Input: part model. Units: mm. Frame: model coordinates. Face numbers are marked on the shaded views. Round coordinates to 2 decimals unless told otherwise and drop trailing zeros. Order: outer loops, then holes, each group sorted by start corner. A loop starts at its lowest first (then second) coordinate and runs counter-clockwise, first axis right, second up. Notation, with made-up numbers: (-30.75, -10.5) -> (8.25, -10.5) arc R20 ccw to (8.25, -2.5) -> close; hole circle Ø9 at (-17, 66.25). An arc over 180 degrees is marked (long way). Use a Markdown table: item, result.
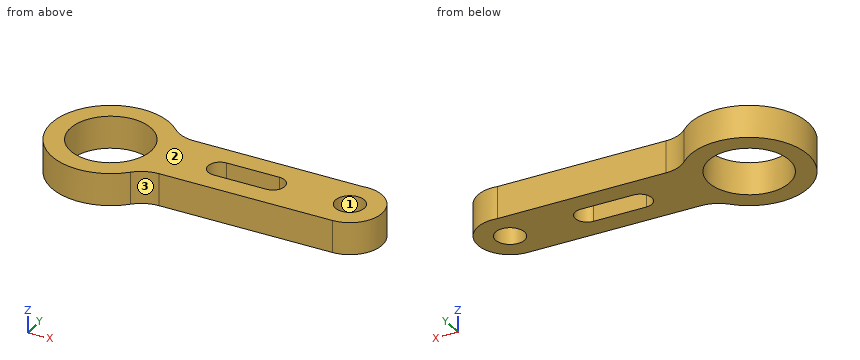
from build123d import *

# Parameters (mm, degrees)
ESQUISSE6_R        = 1.35
ESQUISSE6_R_2      = 3.75
BOSS_EXTRU_6_DEPTH = 3


with BuildPart() as part:
    # Esquisse6 → Boss.-Extru.6 (new body)
    with BuildSketch(Plane.XY):
        with BuildLine():
            Line((-3.987977269, 18.466237455), (-19.940968623, 18.463296912))
            ThreePointArc((-19.940968623, 18.463296912), (-21.090441726, 18.234116339), (-22.064368184, 17.581981843))
            ThreePointArc((-22.064368184, 17.581981843), (-31.458280506, 21.468938246), (-22.060555312, 25.346666961))
            ThreePointArc((-22.060555312, 25.346666961), (-21.088444228, 24.694065374), (-19.940566739, 24.46327096))
            Line((-19.940566739, 24.46327096), (-4.439636922, 24.432043174))
            ThreePointArc((-4.439636922, 24.432043174), (-0.996538054, 21.692713553), (-3.987977269, 18.466237455))
        make_face()
        with Locations((-3.987977269, 21.466237455)):
            Circle(ESQUISSE6_R, mode=Mode.SUBTRACT)
        with Locations((-25.958281169, 21.466237455)):
            Circle(ESQUISSE6_R_2, mode=Mode.SUBTRACT)
        with BuildLine():
            Line((-15.92195018, 22.566237455), (-11.068355584, 22.566237455))
            ThreePointArc((-11.068355584, 22.566237455), (-9.968355584, 21.466237455), (-11.068355584, 20.366237455))
            Line((-11.068355584, 20.366237455), (-15.92195018, 20.366237455))
            ThreePointArc((-15.92195018, 20.366237455), (-17.02195018, 21.466237455), (-15.92195018, 22.566237455))
        make_face(mode=Mode.SUBTRACT)
    extrude(amount=BOSS_EXTRU_6_DEPTH)


solid = part.part
1) Cut plane A-A on x = -23. Return loops of the section in (y, z).
Answer key:
| item | result |
|---|---|
| outline | (16.83, 0) -> (19.16, 0) -> (19.16, 3) -> (16.83, 3) -> close; (23.77, 0) -> (26.1, 0) -> (26.1, 3) -> (23.77, 3) -> close |
2) Ray query, probe 1 along X at (y, z) = (21.5, 1.55); probe 2 along X at (y, z) = (20.5, 0.6); probe 3 along Y at (x, z) = (-4.5, 0.6). Return the intervals inside material, ascending.
Answer key:
| item | result |
|---|---|
| probe 1 | x = -31.46 to -29.71, -22.21 to -17.02, -9.97 to -5.34, -2.64 to -0.99 |
| probe 2 | x = -31.37 to -29.58, -22.33 to -16.45, -10.54 to -4.93, -3.05 to -1.15 |
| probe 3 | y = 18.47 to 20.22, 22.72 to 24.43 |
3) Draft query along X for the marked faces 1, 2 and 3. Return one class per face: released by +X, released by -X, zero draft, split by the parting line, or undercut.
Answer key:
| item | result |
|---|---|
| face 1 | undercut |
| face 2 | zero draft |
| face 3 | released by +X |
4) Cut plane B-B on z = 0.45. Return loops of the section in (x, y), and give its area (3 significant figures).
Answer key:
| item | result |
|---|---|
| outline | (-22.06, 17.58) arc R3 cw to (-19.94, 18.46) -> (-3.99, 18.47) arc R3 ccw (long way) to (-4.44, 24.43) -> (-19.94, 24.46) arc R3 cw to (-22.06, 25.35) arc R5.5 ccw (long way) to start; hole circle Ø7.5 at (-25.96, 21.47); hole (-15.92, 20.37) -> (-11.07, 20.37) arc R1.1 ccw to (-11.07, 22.57) -> (-15.92, 22.57) arc R1.1 ccw to start; hole circle Ø2.7 at (-3.99, 21.47) |
| area | 146 mm^2 |
5) Cut plane C-C on x = -28. Return loops of the section in (y, z), and give its area (3 significant figures).
Answer key:
| item | result |
|---|---|
| outline | (16.36, 0) -> (18.32, 0) -> (18.32, 3) -> (16.36, 3) -> close; (24.61, 0) -> (26.57, 0) -> (26.57, 3) -> (24.61, 3) -> close |
| area | 11.8 mm^2 |
6) Cut plane D-D on y = 16.75. Return loops of the section in (x, z), and give its area (3 significant figures).
Answer key:
| item | result |
|---|---|
| outline | (-28.79, 0) -> (-23.13, 0) -> (-23.13, 3) -> (-28.79, 3) -> close |
| area | 17.0 mm^2 |
7) Contact query for flat-ended pins moving along their axis: P1, Ø1.6, axis at x = -3.99, y = 21.47, coming from the +Z side; P2, Ø1, axis at x = -24.5, z = 1, coming from the -Y side; P3, Ø0.9, axis at x = -14, z = 2, coming from the +Y side. Output: stop coordinate, or through.
Answer key:
| item | result |
|---|---|
| P1 | passes through |
| P2 | stops at y = 16.05 |
| P3 | stops at y = 24.45 |
